from build123d import *

# Parameters (mm, degrees)
BOSS_EXTRUDE1_DEPTH      = 6.35
BOSS_EXTRUDE1_DEPTH_BACK = 6.35
SKETCH1_R                = 3.175


with BuildPart() as part:
    # Sketch1 → Boss-Extrude1 (new, two sides: drawn at the far end of the back side and taken through both)
    with BuildSketch(Plane.XY.offset(-BOSS_EXTRUDE1_DEPTH_BACK)):
        with BuildLine():
            Line((-60.003481739, 12.679905588), (-60.003481739, 50.779905588))
            ThreePointArc((-60.003481739, 50.779905588), (-50.478481739, 60.304905588), (-40.953481739, 50.779905588))
            Line((-40.953481739, 50.779905588), (-40.953481739, 12.679905588))
            Line((-40.953481739, 12.679905588), (-60.003481739, 12.679905588))
        make_face()
        with Locations((-50.478481739, 50.779905588)):
            Circle(SKETCH1_R, mode=Mode.SUBTRACT)
    extrude(amount=BOSS_EXTRUDE1_DEPTH + BOSS_EXTRUDE1_DEPTH_BACK)


solid = part.part
Build history of the part. All positions in model axes, mm. Give positions to 0.01 mm unless a question says otherwise; leave off trailing zeros. Order: outer loops, then holes, each group sorted by start corner. A loop starts at its lowest first (then second) coordinate and runs counter-clockwise, first axis right, second up. Notation, with made-up numbers: M -11,-17.5 L -2,-17.5 A15 cw -2,-5.5 Z; hole C -35.75,16 d4. An arc over 180 degrees is marked long. Use one line per item in the form item = value.
Q1. Slice it at D-D, the plane x = -42.25. Write the cut outline in (y, z), and give its area (3 significant figures).
Conclusion:
outline = M 12.68,-6.35 L 55.58,-6.35 L 55.58,6.35 L 12.68,6.35 Z
area = 545 mm2
Q2. Pull direction X, two halves, no side cores. Call faces 1 (the flat face through (-50, 37, 6.35)), 2 (the cylindrical face through (-49.013, 47.963, -0.089)), 3 (the flat face through (-60.003, 31, 0)): released by +X, released by -X, zero draft, split by the parting line, or undercut.
Conclusion:
face_1 = zero draft
face_2 = undercut
face_3 = released by -X
Q3. Slice it at C-C, the plane z = -0.75. Write the cut outline in (x, y) (3 decimals).
Conclusion:
outline = M -60.003,12.68 L -40.953,12.68 L -40.953,50.78 A9.525 ccw -60.003,50.78 Z; hole C -50.478,50.78 d6.35
Q4. Slice it at A-A, the plane y = 49.5. Write the cut outline in (x, z).
Conclusion:
outline = M -60,-6.35 L -53.38,-6.35 L -53.38,6.35 L -60,6.35 Z; M -47.57,-6.35 L -40.95,-6.35 L -40.95,6.35 L -47.57,6.35 Z
Q5. Wall check: probe 1 along Y at (x, z) = (-50.5, 4); probe 2 along Y at (x, z) = (-52, -5); probe 3 along Y at (x, z) = (-54.5, 3.75). Give the ranges that are in metal, low to high.
Conclusion:
probe_1 = 12.68 to 47.6, 53.95 to 60.3
probe_2 = 12.68 to 47.99, 53.57 to 60.18
probe_3 = 12.68 to 59.41
Q6. Slice it at B-B, the plane x = -49.75. Write the cut outline in (y, z).
Conclusion:
outline = M 12.68,-6.35 L 47.69,-6.35 L 47.69,6.35 L 12.68,6.35 Z; M 53.87,-6.35 L 60.28,-6.35 L 60.28,6.35 L 53.87,6.35 Z
